Verification items for this drawing (mm, ordinates from the low corner). A direction names the side the tool comes from. Coordinates: 2 decimals unless noted, no trailing zeros. Write each loop counter-clockwise with the first axis right and the second up, starting at its lowest first coordinate (ties: lowest second). Pieces come first, ordered by that corner, then holes. Notation, with made-up numbers: (-39, 51) -> (-23, 51) arc R29 cw to (-23, 74) -> close; hole circle Ø10 at (-36, -23.75). An arc over 180 degrees is marked (long way). One line per item, written item: value. Start each with the question number.
1) Gauge pin test, flat ends, axial feed: P1, Ø4, axis at x = 4, z = 6.5, coming from the -Y side; P2, Ø2, axis at x = 9.5, y = 10.5, coming from the -Z side; P3, Ø1, axis at x = 13, z = 4.5, coming from the +Y side. Record the tip position at first contact, or that the pin passes through.
2) Draft check along X on the marked faces 1, 2, 3 and 4. Enter one of: +X half, -X half, draft (parallel to the pull), parting line (faces both ways), or undercut.
3) Set-up check for the marked faces 5 and 6: record each of +Z, -Z, +X, -X, +Y, -Y from which the full face is reachable in a straight line by a thin tool's end or side.
4) Sectioned sample at D-D on x = 1.75. Enter the section's corners in (y, z), plus the area to 3 significant figures.
5) Sectioned sample at A-A on y = 6. Enter the section's corners in (x, z), plus the area to 3 significant figures.
6) Scan lines: line 1 along X through (y, z) = (2.25, 10); line 2 along Y through (x, z) = (12, 6.25); line 3 along Z through (x, y) = (5.5, 6.5). Record each from-to range of solid material in increasing order. Write a range as [from, to].
7) Sectioned sample at C-C on z = 1.5. Enter the section's corners in (x, y).
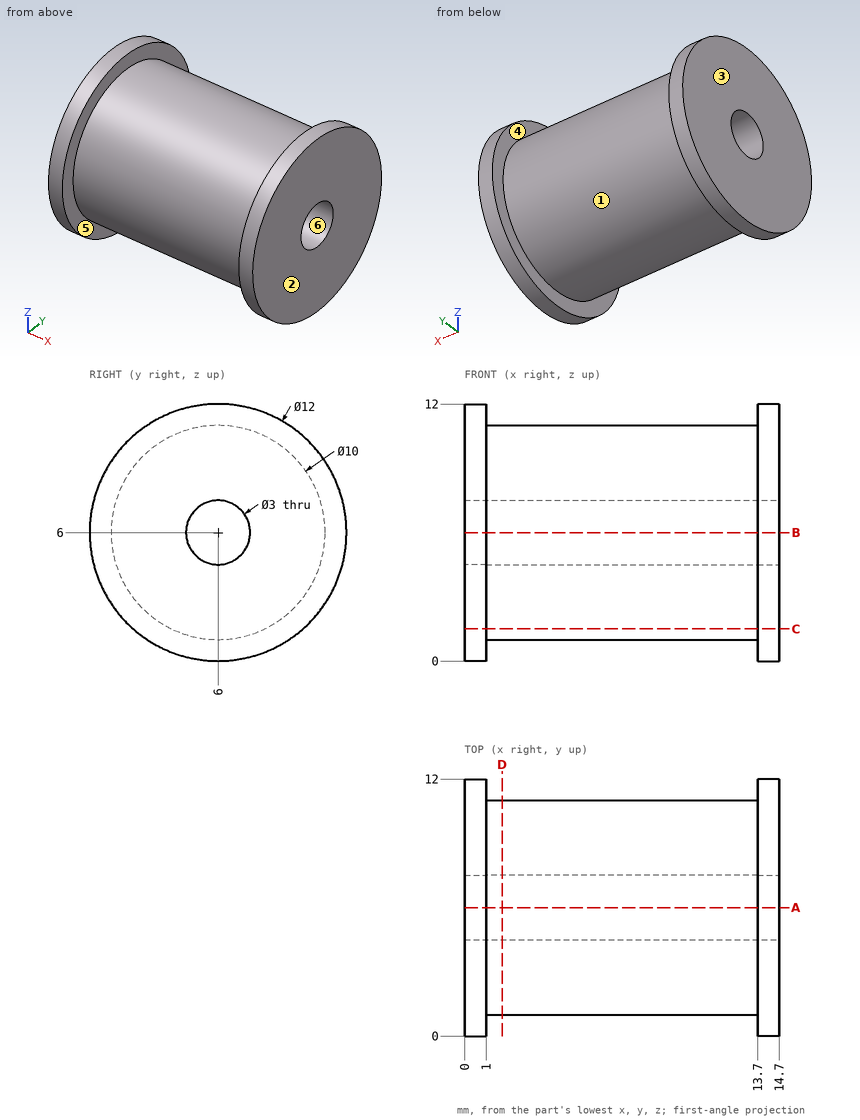
Answers:
1. P1: stops at y = 1
1. P2: stops at z = 2.43
1. P3: stops at y = 10.9
2. face 1: undercut
2. face 2: +X half
2. face 3: -X half
2. face 4: undercut
3. face 5: none
3. face 6: +X, -X
4. outline: circle Ø10 at (6, 6); hole circle Ø3 at (6, 6)
4. area: 71.5 mm2
5. outline: (0, 0) -> (1, 0) -> (1, 1) -> (13.7, 1) -> (13.7, 0) -> (14.7, 0) -> (14.7, 4.5) -> (0, 4.5) -> close; (0, 7.5) -> (14.7, 7.5) -> (14.7, 12) -> (13.7, 12) -> (13.7, 11) -> (1, 11) -> (1, 12) -> (0, 12) -> close
5. area: 107 mm2
6. line 1: x = [0, 1], [13.7, 14.7]
6. line 2: y = [1.01, 4.52], [7.48, 10.99]
6. line 3: z = [1.03, 4.59], [7.41, 10.97]
7. outline: (0, 2.03) -> (1, 2.03) -> (1, 3.82) -> (13.7, 3.82) -> (13.7, 2.03) -> (14.7, 2.03) -> (14.7, 9.97) -> (13.7, 9.97) -> (13.7, 8.18) -> (1, 8.18) -> (1, 9.97) -> (0, 9.97) -> close
